Source: CAD feature listing. Evaluate the final solid. Frame: model axes, mm. Round coordinates to 2 decimals unless told otherwise and drop trailing zeros. Loops run counter-clockwise (first coordinate to the right, second up) from the corner with the lowest first, then second, coordinate; pieces in that order, holes last. Notation, with made-up numbers: (-10, 44) -> (47, 44) arc R27 ccw to (47, 81) -> close; hole circle Ø10 at (-18.75, -10). An arc over 180 degrees is marked (long way). Put each result on its own line as item: value. Start each with the question number.
1. Cut plane A-A (z = 27). Return the cut outline in (x, y).
2. Contact query for flat-ended pins moving along their axis: pin 1 (4 mm diameter, centred on y = 4.5, z = 33, fed in from +X); pin 2 (1.5 mm diameter, centred on y = 17.5, z = 10.5, fed in from +X). Output: stop coordinate, or through.
3. Material intervals for L1, parallel to Y at x = -25.5, z = -38; L2, parallel to Y at x = -28, z = -34.5; L3, parallel to X at y = 20.75, z = -6.5, sorted ascending.
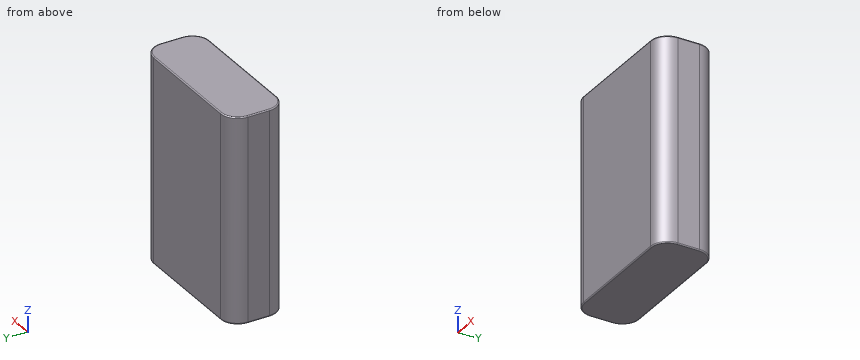
```python
from build123d import *

# Parameters (mm, degrees)
CROQUIS1_W              = 64
CROQUIS1_H              = 90
SALIENTE_EXTRUIR1_DEPTH = 24.5
REDONDEO1_R             = 7.5
REDONDEO2_R             = 0.5


with BuildPart() as part:
    # Croquis1 → Saliente-Extruir1 (new body)
    with BuildSketch(Plane(origin=(0, 0, 0), x_dir=(1, 0, 0), z_dir=(0, 1, 0))):
        Rectangle(CROQUIS1_W, CROQUIS1_H)
    extrude(amount=SALIENTE_EXTRUIR1_DEPTH)

    # Redondeo1
    redondeo1_edges = [part.edges().sort_by_distance(p)[0] for p in [
        (-32, 24.5, 0),
        (32, 24.5, 0),
        (-32, 0, 0),
        (32, 0, 0),
    ]]
    fillet(redondeo1_edges, radius=REDONDEO1_R)

    # Redondeo2
    redondeo2_edges = [part.edges().sort_by_distance(p)[0] for p in [
        (-32, 12.25, 45),
        (-32, 12.25, -45),
        (0, 0, 45),
        (32, 12.25, 45),
        (0, 24.5, 45),
        (29.803300859, 22.303300859, 45),
        (29.803300859, 2.196699141, 45),
        (-29.803300859, 22.303300859, 45),
        (-29.803300859, 2.196699141, 45),
        (0, 0, -45),
        (0, 24.5, -45),
        (32, 12.25, -45),
        (29.803300859, 22.303300859, -45),
        (29.803300859, 2.196699141, -45),
        (-29.803300859, 22.303300859, -45),
        (-29.803300859, 2.196699141, -45),
    ]]
    fillet(redondeo2_edges, radius=REDONDEO2_R)


solid = part.part
```
Solution:
1. outline: (-32, 7.5) arc R7.5 ccw to (-24.5, 0) -> (24.5, 0) arc R7.5 ccw to (32, 7.5) -> (32, 17) arc R7.5 ccw to (24.5, 24.5) -> (-24.5, 24.5) arc R7.5 ccw to (-32, 17) -> close
2. pin 1: stops at x = 31.93
2. pin 2: stops at x = 32
3. L1: y = 0.07 to 24.43
3. L2: y = 0.87 to 23.63
3. L3: x = -31 to 31
